from build123d import *

# Parameters (mm, degrees)
SKETCH_1_W          = 69.6
SKETCH_1_H          = 69.6
SKETCH_1_W_2        = 65.6
SKETCH_1_H_2        = 65.6
EXTRUDE_1_DEPTH     = 8
SKETCH_2_W          = 73.6
SKETCH_2_H          = 73.6
EXTRUDE_2_DEPTH     = 2
SKETCH_3_R          = 0.95
CUT_EXTRUDE_1_DEPTH = 81.899938195
SKETCH_4_R          = 0.95
CUT_EXTRUDE_2_DEPTH = 81.899938195


with BuildPart() as part:
    # 草图1 → 凸台-拉伸1 (new body)
    with BuildSketch(Plane(origin=(0, 0, 0), x_dir=(1, 0, 0), z_dir=(0, 1, 0))):
        Rectangle(SKETCH_1_W, SKETCH_1_H)
        Rectangle(SKETCH_1_W_2, SKETCH_1_H_2, mode=Mode.SUBTRACT)
    extrude(amount=EXTRUDE_1_DEPTH)

    # 草图2 → 凸台-拉伸2 (add)
    with BuildSketch(Plane.XZ):
        Rectangle(SKETCH_2_W, SKETCH_2_H)
        with BuildLine():
            Line((-15, -13), (15, -13))
            ThreePointArc((15, -13), (22, -20), (15, -27))
            Line((15, -27), (-15, -27))
            ThreePointArc((-15, -27), (-22, -20), (-15, -13))
        make_face(mode=Mode.SUBTRACT)
    extrude(amount=EXTRUDE_2_DEPTH)

    # 草图3 → 切除-拉伸1 (cut, through all)
    with BuildSketch(Plane.ZY.offset(34.8)):
        with Locations((17.5, 4)):
            Circle(SKETCH_3_R)
        with Locations((-17.5, 4)):
            Circle(SKETCH_3_R)
    extrude(amount=-CUT_EXTRUDE_1_DEPTH, mode=Mode.SUBTRACT)

    # 草图4 → 切除-拉伸2 (cut, through all)
    with BuildSketch(Plane(origin=(0, 0, -34.8), x_dir=(-1, 0, 0), z_dir=(0, 0, -1))):
        with Locations((17.5, 4)):
            Circle(SKETCH_4_R)
        with Locations((-17.5, 4)):
            Circle(SKETCH_4_R)
    extrude(amount=-CUT_EXTRUDE_2_DEPTH, mode=Mode.SUBTRACT)


solid = part.part
For this review, take the finished solid that the model builds, in its own axes (mm). A direction names the side the tool comes from. Round coordinates to 2 decimals unless told otherwise and drop trailing zeros. Loops run counter-clockwise (first coordinate to the right, second up) from the corner with the lowest first, then second, coordinate; pieces in that order, holes last. Notation, with made-up numbers: (-24, 22) - (29, 22) arc R23 ccw to (29, 58) - close; hole circle Ø5 at (46, -14.75). An arc over 180 degrees is marked (long way). Put each result on its own line as item: value. Start each with the question number.
1. Consider section C-C on x = -29.5. State the section outline as (y, z) points.
2. Consider section B-B on z = 17.5. State the section outline as (x, y) points, plus the area to 3 significant figures.
3. Consider section D-D on y = 2. State the section outline as (x, z) points.
4. Consider section A-A on z = -20. State the section outline as (x, y) points.
5. For probe 1 along X at (y, z) = (2.75, -13.5); probe 2 along Y at (x, z) = (-33.95, 17.5); probe 3 along X at (y, z) = (-0.5, -20), list the stretches that pass through material, from the lowest coordinate up. Write a range as [from, to].
6. Mouldability with a two-part tool opening along Y and no side actions: class faces 4 (the flat face through (-1, -2, 1)), 5 (the flat face through (-3, 8, 33)), 6 (the cylindrical face through (-33.81, 3.64, -16.62)) as +Y half, -Y half, draft (parallel to the pull), parting line (faces both ways), or undercut.
7. Insertion check: P1, Ø4, axis at y = 5.5, z = -17.5, coming from the -X side; P2, Ø1.5, axis at x = 28, z = 24, coming from the +Y side; P3, Ø5, axis at y = 7, z = 5, coming from the +X side. Each pin has a flat end and moves straight along its axis. Give the tip position at first contact, or say it passes through.
8. For faces 1 (the flat face through (34.8, 4, 0)), 2 (the flat face through (0, 4, -32.8)), 3 (the cylindrical face through (22, -1, -20)), list the 3-axis set-ups (+Z, -Z, +X, -X, +Y, -Y) from which the entire face can be reached by the end or side of a thin tool; tool diameter is ignored.
Result sheet:
1. outline: (-2, -36.8) - (0, -36.8) - (0, -34.8) - (8, -34.8) - (8, -32.8) - (0, -32.8) - (0, 32.8) - (8, 32.8) - (8, 34.8) - (0, 34.8) - (0, 36.8) - (-2, 36.8) - close
2. outline: (-36.8, -2) - (36.8, -2) - (36.8, 0) - (34.8, 0) - (34.8, 3.05) - (32.8, 3.05) - (32.8, 0) - (-32.8, 0) - (-32.8, 3.05) - (-34.8, 3.05) - (-34.8, 0) - (-36.8, 0) - close; (-34.8, 4.95) - (-32.8, 4.95) - (-32.8, 8) - (-34.8, 8) - close; (32.8, 4.95) - (34.8, 4.95) - (34.8, 8) - (32.8, 8) - close
2. area: 172 mm^2
3. outline: (-34.8, -34.8) - (34.8, -34.8) - (34.8, 34.8) - (-34.8, 34.8) - close; hole (-32.8, -32.8) - (32.8, -32.8) - (32.8, 32.8) - (-32.8, 32.8) - close
4. outline: (-36.8, -2) - (-22, -2) - (-22, 0) - (-32.8, 0) - (-32.8, 8) - (-34.8, 8) - (-34.8, 0) - (-36.8, 0) - close; (22, -2) - (36.8, -2) - (36.8, 0) - (34.8, 0) - (34.8, 8) - (32.8, 8) - (32.8, 0) - (22, 0) - close
5. probe 1: [-34.8, -32.8], [32.8, 34.8]
5. probe 2: [-2, 3.05], [4.95, 8]
5. probe 3: [-36.8, -22], [22, 36.8]
6. face 4: -Y half
6. face 5: +Y half
6. face 6: undercut
7. P1: x = -34.8
7. P2: y = 0
7. P3: x = 34.8
8. face 1: +Z, -Z, +X, +Y
8. face 2: +Y
8. face 3: +Y, -Y
